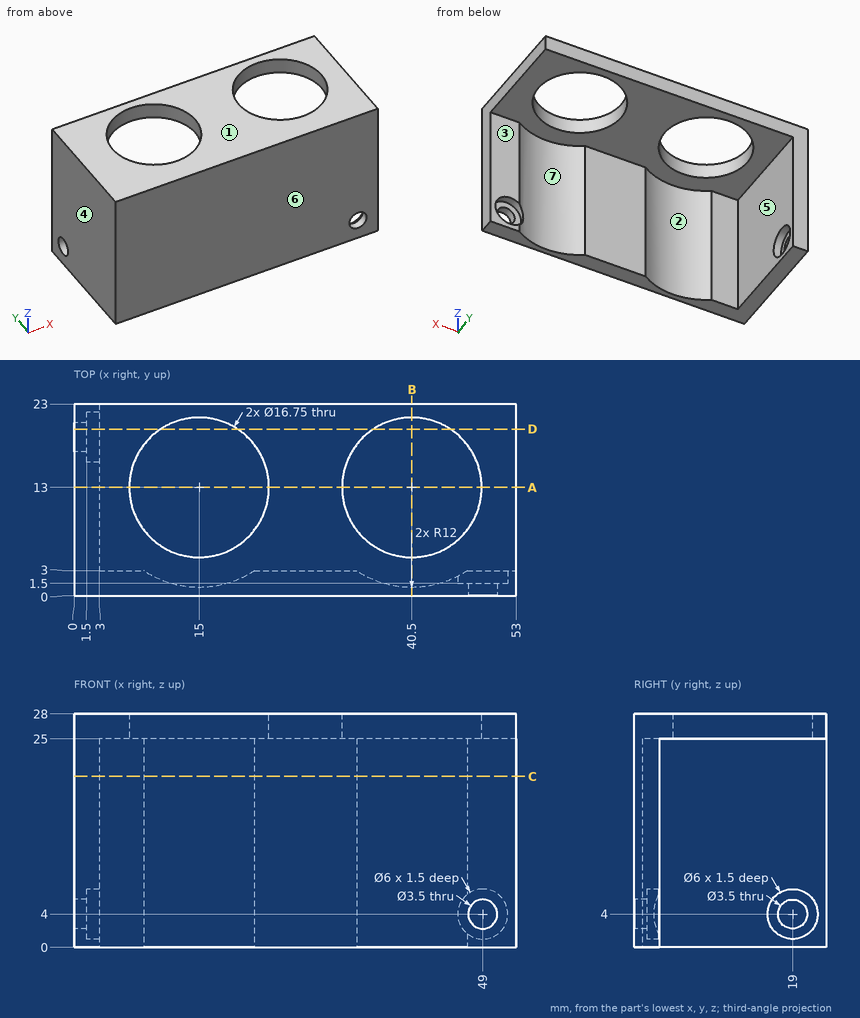
Job drawing, mm, ordinate dimensions from the low corner. One solid piece. A direction names the side the tool comes from. Give positions to 0.01 mm unless a question says otherwise; leave off trailing zeros. Order: outer loops, then holes, each group sorted by start corner. A loop starts at its lowest first (then second) coordinate and runs counter-clockwise, first axis right, second up. Notation, with made-up numbers: M -20.75,2 L -10.75,2 A34 ccw -10.75,38 Z; hole C 54,42 d5. An arc over 180 degrees is marked long. Put each result on its own line as item: value. Start each with the question number.
(1) Tool access for the marked faces 1, 2 and 3: list every direction of +Z, -Z, +X, -X, +Y, -Y with a clear straight run to the whole face (end or side of a thin tool).
(2) Pull direction X, two halves, no side cores. Call the marked faces 4, 5, 6 and 7: released by +X, released by -X, zero draft, split by the parting line, or undercut.
(3) Band-saw the part on C-C on z = 20.5. Give the cut face in (x, y).
(4) Pin check, flat tips, straight feed: pin 1 Ø6.5 at (x, z) = (51, 10) entering from +Y; pin 2 Ø1 at (x, y) = (27, 8.5) entering from -Z; pin 3 Ø1.8 at (y, z) = (20, 3) entering from +X; pin 4 Ø1.8 at (x, z) = (48.5, 4.5) entering from +Y. Stop position of each tip, or through.
(5) Band-saw the part on B-B on x = 40.5. Give the cut face in (y, z) (3 decimals).
(6) Drill centre lines: L1, parallel to Y at x = 15, z = 27 (3 decimals); L2, parallel to X at y = 2.2, z = 4; L3, parallel to Z at x = 0.3, y = 19. Where is each one in solid material? Low to high. Write a range as [from, to].
(7) Band-saw the part on D-D on y = 20. Give the cut face in (x, z).
(8) Band-saw the part on A-A on y = 13. Give the cut face in (x, z) (3 decimals), then the cut area to 4 significant figures.
Results below:
1. face 1: +Z, +X, -X, +Y, -Y
1. face 2: -Z, +Y
1. face 3: -Z, +X, +Y
2. face 4: released by -X
2. face 5: released by +X
2. face 6: zero draft
2. face 7: undercut
3. outline: M 0,0 L 53,0 L 53,3 L 47.13,3 A12 cw 33.87,3 L 21.63,3 A12 cw 8.37,3 L 3,3 L 3,23 L 0,23 Z
4. pin 1: stops at y = 3
4. pin 2: stops at z = 25
4. pin 3: stops at x = 1.5
4. pin 4: passes through
5. outline: M 0,0 L 1,0 L 1,25 L 4.625,25 L 4.625,28 L 0,28 Z; M 21.375,25 L 23,25 L 23,28 L 21.375,28 Z
6. L1: y = [0, 4.625], [21.375, 23]
6. L2: x = [0, 9.77], [20.23, 35.27], [45.73, 46], [52, 53]
6. L3: z = [0, 2.25], [5.75, 28]
7. outline: M 0,0 L 3,0 L 3,1.17 L 1.5,1.17 L 1.5,2.56 L 0,2.56 Z; M 0,5.44 L 1.5,5.44 L 1.5,6.83 L 3,6.83 L 3,25 L 10.4,25 L 10.4,28 L 0,28 Z; M 19.6,25 L 35.9,25 L 35.9,28 L 19.6,28 Z; M 45.1,25 L 53,25 L 53,28 L 45.1,28 Z
8. outline: M 0,0 L 3,0 L 3,25 L 6.625,25 L 6.625,28 L 0,28 Z; M 23.375,25 L 32.125,25 L 32.125,28 L 23.375,28 Z; M 48.875,25 L 53,25 L 53,28 L 48.875,28 Z
8. area: 133.5 mm2
